Can you work these out from the model? Positions are in its coordinate system, mm. Give positions to 0.01 mm unless a question says otherwise; leave off trailing zeros. Loops run counter-clockwise (first coordinate to the right, second up) from the corner with the lowest first, then second, coordinate; pieces in that order, holes last. Notation, with made-up numbers: (-4, 74) -> (7, 74) arc R34 cw to (7, 104) -> close; hole circle Ø7 at (9.25, -35). An arc over 180 degrees is marked (long way). Use CSV: the item, a comma, the result in double quotes.
Autodesk Inventor part; units mm, degrees
ref_plane "YZ Plane" through (0, 0, 0) normal (1, 0, 0) x (0, 1, 0)
ref_plane "XZ Plane" through (0, 0, 0) normal (0, 1, 0) x (-1, 0, 0)
ref_plane "XY Plane" through (0, 0, 0) normal (0, 0, 1) x (1, 0, 0)
sketch "Sketch1" plane through (0, 0, 0) normal (0, 0, 1) x (1, 0, 0)
  line L0 (-190.5, 50.8) -> (190.5, 50.8)
  line L1 (190.5, 50.8) -> (190.5, -50.8)
  line L2 (115.8875, -50.8) -> (-115.8875, -50.8)
  line L3 (-190.5, -50.8) -> (-190.5, 50.8)
  line L4 (-190.5, 50.8) -> (190.5, -50.8) construction
  line L5 (190.5, 50.8) -> (-190.5, -50.8) construction
  circle A0 centre (-127, 10.16) radius 9.525
  circle A1 centre (-109.0422, 28.1178) radius 2.3812
  circle A2 centre (-144.9578, -7.7978) radius 2.3812
  line L6 (0, 0) -> (0, 83.7438) construction
  circle A3 centre (127, 10.16) radius 9.525
  circle A4 centre (109.0422, 28.1178) radius 2.3812
  circle A5 centre (144.9578, -7.7978) radius 2.3812
  line L7 (115.8875, -50.8) -> (115.8875, -152.4)
  line L8 (-190.5, -50.8) -> (-190.5, -152.4)
  line L9 (190.5, -50.8) -> (190.5, -152.4)
  line L10 (-190.5, -152.4) -> (-115.8875, -152.4)
  line L11 (115.8875, -152.4) -> (190.5, -152.4)
  line L12 (-115.8875, -27.9247) -> (-115.8875, -30.9033)
  line L13 (-115.8875, -50.8) -> (-115.8875, -152.4)
  dimension "d0" = 381
  dimension "d1" = 101.6
  dimension "d2" = 19.05
  dimension "d4" = 127
  dimension "d5" = 60.96
  dimension "d6" = 4.7625
  dimension "d8" = 17.9578
  dimension "d9" = 17.9578
  dimension "d10" = 4.7625
  dimension "d11" = 17.9578
  dimension "d12" = 17.9578
  dimension "d15" = 115.8875
extrude "Extrusion1" add sketch "Sketch1" along normal mid plane 11.999
properties part number "Indexer Upper Plate"
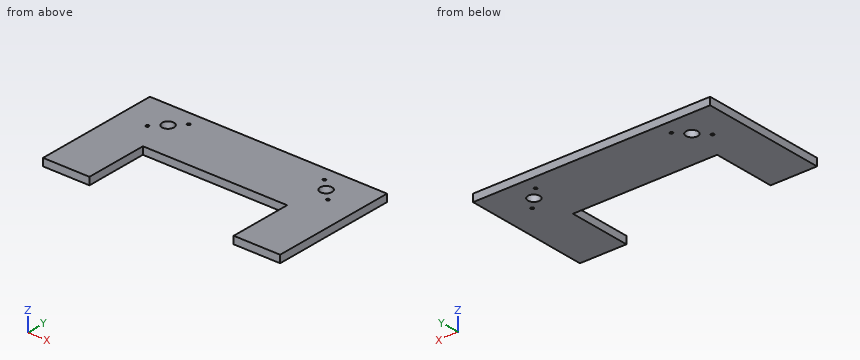
(1) If I drill on L1, parallel to Y at x = 109.5, z = -1.5; L2, parallel to X at y = -113, z = 4.75; L3, parallel to Y at x = 127, z = -1.25 (3 decimals), over which ranges is the centre line in solid material (lowest first)? Write a range as from..to.
Answer sheet:
L1,"y = -50.8..25.78, 30.45..50.8"
L2,"x = -190.5..-115.89, 115.89..190.5"
L3,"y = -152.4..0.635, 19.685..50.8"
(2) If we section it at B-B, the plane x = -127: Write out the boundary of the cut face in (y, z) (1 decimal).
Answer sheet:
outline,"(-152.4, -6) -> (0.6, -6) -> (0.6, 6) -> (-152.4, 6) -> close; (19.7, -6) -> (50.8, -6) -> (50.8, 6) -> (19.7, 6) -> close"
(3) Will this pin go through, and if not, where does the flat tip stop? pin 1 Ø3.5 at (x, z) = (-57.5, -2) entering from -Y.
Answer sheet:
pin 1,"stops at y = -50.8"
(4) If we section it at C-C, the plane y = 10.16: Write out the boundary of the cut face in (x, z) (1 decimal).
Answer sheet:
outline,"(-190.5, -6) -> (-136.5, -6) -> (-136.5, 6) -> (-190.5, 6) -> close; (-117.5, -6) -> (117.5, -6) -> (117.5, 6) -> (-117.5, 6) -> close; (136.5, -6) -> (190.5, -6) -> (190.5, 6) -> (136.5, 6) -> close"
(5) If we section it at A-A, the plane y = -56.5: Write out the boundary of the cut face in (x, z), then the cut area to 3 significant figures.
Answer sheet:
outline,"(-190.5, -6) -> (-115.89, -6) -> (-115.89, 6) -> (-190.5, 6) -> close; (115.89, -6) -> (190.5, -6) -> (190.5, 6) -> (115.89, 6) -> close"
area,"1,790 mm2"
(6) If we section it at D-D, the plane z = 0.25: Give the number of separate pieces and of enclosed holes in the cut face, then the cut area to 3 significant figures.
Answer sheet:
separate pieces,"1"
enclosed holes,"6"
area,"53,200 mm2"
